For this review, take the finished solid that the model builds, in its own axes (mm). Give positions to 0.01 mm unless a question says otherwise; leave off trailing zeros. Loops run counter-clockwise (first coordinate to the right, second up) from the corner with the lowest first, then second, coordinate; pieces in that order, holes last.
```python
from build123d import *

# Parameters (mm, degrees)
BOSS_EXTRUDE1_DEPTH = 1
SKETCH5_W           = 0.5
SKETCH5_H           = 0.5
BOSS_EXTRUDE2_DEPTH = 25


with BuildPart() as part:
    # Sketch1 → Boss-Extrude1 (new body)
    with BuildSketch(Plane(origin=(0, 0, 0), x_dir=(1, 0, 0), z_dir=(0, 1, 0))):
        with BuildLine():
            Line((2.525, -1.573213272), (2.525, 1.573213272))
            ThreePointArc((2.525, 1.573213272), (-2.975, 0), (2.525, -1.573213272))
        make_face()
    extrude(amount=BOSS_EXTRUDE1_DEPTH)

    # Sketch4 → Revolve1 (revolve)
    with BuildSketch(Plane.XY):
        with BuildLine():
            Line((-2.475, 1), (-2.475, 5.875))
            ThreePointArc((-2.475, 5.875), (-1.750089283, 7.625089283), (0, 8.35))
            Line((0, 8.35), (0, 1))
            Line((0, 1), (-2.475, 1))
        make_face()
    revolve(axis=Axis((0, 0, 0), (0, 1, 0)))

    # Sketch5 → Boss-Extrude2 (add)
    with BuildSketch(Plane(origin=(0, 0, 0), x_dir=(-1, 0, 0), z_dir=(0, -1, 0))):
        with Locations((-1.2, 0)):
            Rectangle(SKETCH5_W, SKETCH5_H)
        with Locations((1.2, 0)):
            Rectangle(SKETCH5_W, SKETCH5_H)
    extrude(amount=BOSS_EXTRUDE2_DEPTH)


solid = part.part
```
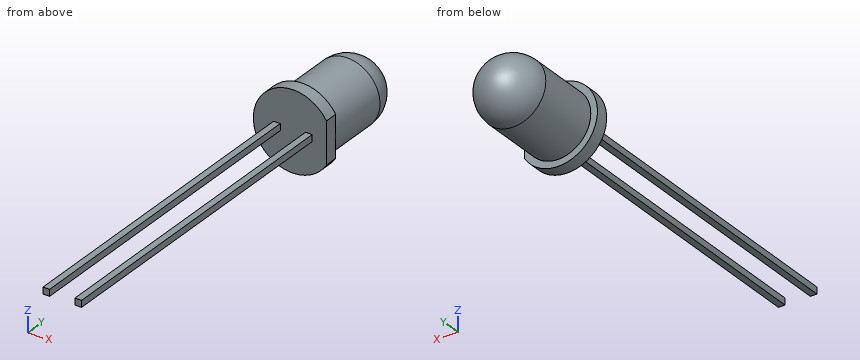
Q1. Consider section C-C on z = -2.2. Give the boundary of the cut face in (x, y) (3 decimals).
Answers:
outline: (-2.003, 0) - (2.003, 0) - (2.003, 1) - (1.134, 1) - (1.134, 5.875) arc R1.134 ccw to (-1.134, 5.875) - (-1.134, 1) - (-2.003, 1) - close
Q2. For probe 1 along Z at (x, y) = (1.3, -14); probe 2 along Y at (x, z) = (1.55, 2.25); probe 3 along Z at (x, y) = (-0.1, 5.5), list the stretches that pass through material, from the lowest coordinate up.
Answers:
probe 1: z = -0.25 to 0.25
probe 2: y = 0 to 1
probe 3: z = -2.47 to 2.47
Q3. Consider section A-A on y = -1. Give the boundary of the cut face in (x, z), plus the area to 3 significant figures.
Answers:
outline: (-1.45, -0.25) - (-0.95, -0.25) - (-0.95, 0.25) - (-1.45, 0.25) - close; (0.95, -0.25) - (1.45, -0.25) - (1.45, 0.25) - (0.95, 0.25) - close
area: 0.500 mm2
Q4. For pin 1 Ø2 at (x, z) = (2, -2) entering from -Y; pin 2 Ø0.6 at (x, y) = (-1, -13) entering from -Z; pin 3 Ø0.6 at (x, y) = (1.5, -15.5) entering from +Z, all flat-tipped, find the tip position at first contact; note any pin that passes through.
Answers:
pin 1: stops at y = 0
pin 2: stops at z = -0.25
pin 3: stops at z = 0.25
Q5. Consider section B-B on x = 0. Give the boundary of the cut face in (y, z) (3 decimals).
Answers:
outline: (0, -2.975) - (1, -2.975) - (1, -2.475) - (5.875, -2.475) arc R2.475 ccw to (5.875, 2.475) - (1, 2.475) - (1, 2.975) - (0, 2.975) - close
